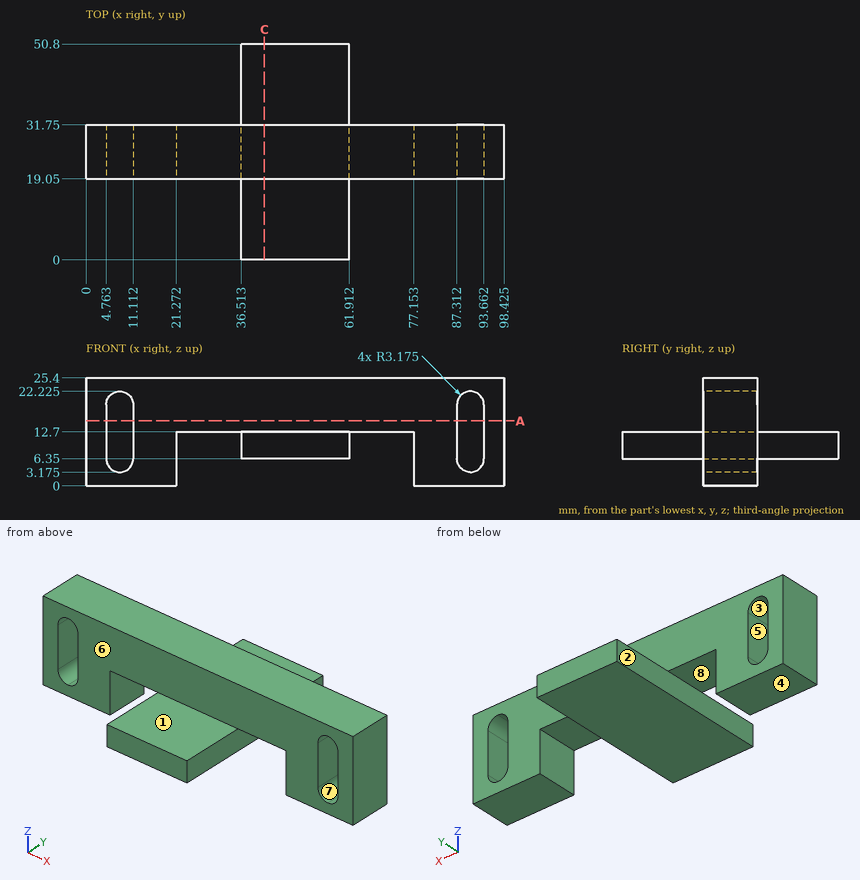
Job drawing, mm, ordinate dimensions from the low corner. One solid piece. A direction names the side the tool comes from. Coordinates: 2 decimals unless noted, no trailing zeros. Order: outer loops, then holes, each group sorted by start corner. A loop starts at its lowest first (then second) coordinate and runs counter-clockwise, first axis right, second up. Notation, with made-up numbers: (70.25, -34.75) -> (108.25, -34.75) arc R30 ccw to (108.25, -8.75) -> close; hole circle Ø9 at (25, 75.5). An arc over 180 degrees is marked (long way). Put each result on its own line as item: value. Start each with the question number.
(1) Which spindle directions (+Z, -Z, +X, -X, +Y, -Y) get a long thin tool onto all of the face, cutting with end or side? Do the marked faces 1, 2, 3 and 4. Say none if no direction does.
(2) Band-saw the part on A-A (z = 15.25). Count the separate pieces of the cut face and the enclosed holes in it, then the cut area to 3 significant figures.
(3) Mould opens along Z. For the marked faces 5, 6, 7 and 8 say: pulls with the +Z half, pulls with the -Z half, needs draft (parallel to the pull), parting line crosses it, or undercut.
(4) Probe line 1 along Z through (x, y) = (59.5, 18.5); line 2 along Z through (x, y) = (26.5, 21); line 3 along Y through (x, z) = (79, 5). List the from-to ranges inside material, lowest first. Write a range as [from, to].
(5) Pin check, flat tips, straight feed: pin 1 Ø1.5 at (x, y) = (53, 11.5) entering from +Z; pin 2 Ø7.5 at (x, y) = (43.5, 34) entering from -Z; pin 3 Ø7.5 at (x, z) = (67, 16) entering from +Y. Stop position of each tip, or through.
(6) Band-saw the part on C-C (x = 42). Give the cut face in (y, z).
Determined:
1. face 1: +Z, +X, -X, -Y
1. face 2: -Z, +Y, -Y
1. face 3: +Y, -Y
1. face 4: -Z, +X, -X, +Y, -Y
2. separate pieces: 3
2. enclosed holes: 0
2. area: 1,090 mm²
3. face 5: undercut
3. face 6: needs draft
3. face 7: undercut
3. face 8: pulls with the -Z half
4. line 1: z = [6.35, 12.7]
4. line 2: z = [12.7, 25.4]
4. line 3: y = [19.05, 31.75]
5. pin 1: stops at z = 12.7
5. pin 2: stops at z = 6.35
5. pin 3: stops at y = 31.75
6. outline: (0, 6.35) -> (50.8, 6.35) -> (50.8, 12.7) -> (31.75, 12.7) -> (31.75, 25.4) -> (19.05, 25.4) -> (19.05, 12.7) -> (0, 12.7) -> close
